Geometry check sheet. Reference: the model listing, model coordinates, mm. A direction names the side the tool comes from. Round coordinates to 2 decimals unless told otherwise and drop trailing zeros. Write each loop counter-clockwise with the first axis right and the second up, starting at its lowest first coordinate (ties: lowest second). Pieces come first, ordered by that corner, then holes. Notation, with made-up numbers: (3.25, -29.75) - (23.25, -29.75) arc R19 ccw to (23.25, -8.75) - close; hole circle Ø11 at (-1.75, 78.5). An arc over 180 degrees is marked (long way). Return JSON: item names as keys, results as strings.
```python
from build123d import *

# Parameters (mm, degrees)
ESQUISSE1_R             = 25.4
BOSS_EXTRU_1_DEPTH      = 25
ESQUISSE6_R             = 1.55
ENL_V_MAT_EXTRU_4_DEPTH = 6
ESQUISSE8_R             = 25.4
BOSS_EXTRU_3_DEPTH      = 10
ESQUISSE9_R             = 1.5
ENL_V_MAT_EXTRU_5_DEPTH = 10


with BuildPart() as part:
    # Esquisse1 → Boss.-Extru.1 (new body)
    with BuildSketch(Plane.XY):
        with Locations((16.625210007, 7.108710486)):
            Circle(ESQUISSE1_R)
    extrude(amount=BOSS_EXTRU_1_DEPTH)

    # Esquisse6 → Enlèv. mat.-Extru.4 (cut)
    with BuildSketch(Plane(origin=(0, 0, 0), x_dir=(-1, 0, 0), z_dir=(0, 0, -1))):
        with Locations((-39.525210007, 7.108710486)):
            Circle(ESQUISSE6_R)
        with Locations((6.274789993, 7.108710486)):
            Circle(ESQUISSE6_R)
    extrude(amount=-ENL_V_MAT_EXTRU_4_DEPTH, mode=Mode.SUBTRACT)

    # Esquisse8 → Boss.-Extru.3 (add)
    with BuildSketch(Plane.XY.offset(25)):
        with Locations((16.625210007, 7.108710486)):
            Circle(ESQUISSE8_R)
    extrude(amount=BOSS_EXTRU_3_DEPTH)

    # Esquisse9 → Enlèv. mat.-Extru.5 (cut)
    with BuildSketch(Plane.XY.offset(35)):
        with Locations((16.625210007, 7.108710486)):
            Circle(ESQUISSE9_R)
        with Locations((21.905210007, 7.108710486)):
            Circle(ESQUISSE9_R)
        with Locations((27.185210007, 7.108710486)):
            Circle(ESQUISSE9_R)
        with Locations((32.465210007, 7.108710486)):
            Circle(ESQUISSE9_R)
        with Locations((37.745210007, 7.108710486)):
            Circle(ESQUISSE9_R)
        with Locations((11.345210007, 7.108710486)):
            Circle(ESQUISSE9_R)
        with Locations((6.065210007, 7.108710486)):
            Circle(ESQUISSE9_R)
        with Locations((0.785210007, 7.108710486)):
            Circle(ESQUISSE9_R)
        with Locations((-4.494789993, 7.108710486)):
            Circle(ESQUISSE9_R)
        with Locations((0.785210007, 17.668710486)):
            Circle(ESQUISSE9_R)
        with Locations((6.065210007, 17.668710486)):
            Circle(ESQUISSE9_R)
        with Locations((11.345210007, 17.668710486)):
            Circle(ESQUISSE9_R)
        with Locations((16.625210007, 17.668710486)):
            Circle(ESQUISSE9_R)
        with Locations((21.905210007, 17.668710486)):
            Circle(ESQUISSE9_R)
        with Locations((27.185210007, 17.668710486)):
            Circle(ESQUISSE9_R)
        with Locations((32.465210007, 17.668710486)):
            Circle(ESQUISSE9_R)
        with Locations((8.705210007, 12.388710486)):
            Circle(ESQUISSE9_R)
        with Locations((13.985210007, 12.388710486)):
            Circle(ESQUISSE9_R)
        with Locations((19.265210007, 12.388710486)):
            Circle(ESQUISSE9_R)
        with Locations((24.545210007, 12.388710486)):
            Circle(ESQUISSE9_R)
        with Locations((29.825210007, 12.388710486)):
            Circle(ESQUISSE9_R)
        with Locations((35.105210007, 12.388710486)):
            Circle(ESQUISSE9_R)
        with Locations((3.425210007, 12.388710486)):
            Circle(ESQUISSE9_R)
        with Locations((-1.854789993, 12.388710486)):
            Circle(ESQUISSE9_R)
        with Locations((13.985210007, 22.948710486)):
            Circle(ESQUISSE9_R)
        with Locations((19.265210007, 22.948710486)):
            Circle(ESQUISSE9_R)
        with Locations((24.545210007, 22.948710486)):
            Circle(ESQUISSE9_R)
        with Locations((13.985210007, 28.228710486)):
            Circle(ESQUISSE9_R)
        with Locations((19.265210007, 28.228710486)):
            Circle(ESQUISSE9_R)
        with Locations((24.545210007, 28.228710486)):
            Circle(ESQUISSE9_R)
        with Locations((8.705210007, 22.948710486)):
            Circle(ESQUISSE9_R)
        with Locations((8.705210007, 28.228710486)):
            Circle(ESQUISSE9_R)
        with Locations((29.825210007, 22.948710486)):
            Circle(ESQUISSE9_R)
        with Locations((3.425210007, 22.948710486)):
            Circle(ESQUISSE9_R)
        with Locations((35.105210007, 1.828710486)):
            Circle(ESQUISSE9_R)
        with Locations((29.825210007, 1.828710486)):
            Circle(ESQUISSE9_R)
        with Locations((24.545210007, 1.828710486)):
            Circle(ESQUISSE9_R)
        with Locations((19.265210007, 1.828710486)):
            Circle(ESQUISSE9_R)
        with Locations((13.985210007, 1.828710486)):
            Circle(ESQUISSE9_R)
        with Locations((8.705210007, 1.828710486)):
            Circle(ESQUISSE9_R)
        with Locations((3.425210007, 1.828710486)):
            Circle(ESQUISSE9_R)
        with Locations((-1.854789993, 1.828710486)):
            Circle(ESQUISSE9_R)
        with Locations((0.785210007, -3.451289514)):
            Circle(ESQUISSE9_R)
        with Locations((6.065210007, -3.451289514)):
            Circle(ESQUISSE9_R)
        with Locations((11.345210007, -3.451289514)):
            Circle(ESQUISSE9_R)
        with Locations((16.625210007, -3.451289514)):
            Circle(ESQUISSE9_R)
        with Locations((21.905210007, -3.451289514)):
            Circle(ESQUISSE9_R)
        with Locations((27.185210007, -3.451289514)):
            Circle(ESQUISSE9_R)
        with Locations((32.465210007, -3.451289514)):
            Circle(ESQUISSE9_R)
        with Locations((29.825210007, -8.731289514)):
            Circle(ESQUISSE9_R)
        with Locations((24.545210007, -8.731289514)):
            Circle(ESQUISSE9_R)
        with Locations((19.265210007, -8.731289514)):
            Circle(ESQUISSE9_R)
        with Locations((13.985210007, -8.731289514)):
            Circle(ESQUISSE9_R)
        with Locations((8.705210007, -8.731289514)):
            Circle(ESQUISSE9_R)
        with Locations((3.425210007, -8.731289514)):
            Circle(ESQUISSE9_R)
        with Locations((8.705210007, -14.011289514)):
            Circle(ESQUISSE9_R)
        with Locations((13.985210007, -14.011289514)):
            Circle(ESQUISSE9_R)
        with Locations((19.265210007, -14.011289514)):
            Circle(ESQUISSE9_R)
        with Locations((24.545210007, -14.011289514)):
            Circle(ESQUISSE9_R)
    extrude(amount=-ENL_V_MAT_EXTRU_5_DEPTH, mode=Mode.SUBTRACT)

    # Esquisse12 → Enlèvement de matière-Révolution1 (revolve, cut)
    with BuildSketch(Plane(origin=(16.625210007, 0, 0), x_dir=(0, 0, -1), z_dir=(1, 0, 0))):
        Polygon((0, 7.108710486), (0, 27.108710486), (-25, 30.108710486), (-25, 7.108710486), align=None)
    revolve(axis=Axis((16.625210007, 7.108710486, 25), (0, 0, -1)), mode=Mode.SUBTRACT)


solid = part.part
```
(1) Gauge pin test, flat ends, axial feed: pin 1 (1 mm diameter, centred on x = 21.5, z = 13.5, fed in from -Y); pin 2 (4 mm diameter, centred on x = 27.19, y = 17.67, fed in from -Z); pin 3 (4 mm diameter, centred on x = 28, z = 30.5, fed in from -Y); pin 4 (1.8 mm diameter, centred on x = 16.63, y = -3.45, fed in from -Z). Record the tip position at first contact, or that the pin passes through.
Response values:
{"pin 1": "stops at y = -17.91", "pin 2": "stops at z = 25", "pin 3": "stops at y = -16.5", "pin 4": "passes through"}
(2) Release check for a two-part mould opening along X. For faces 4 (the face through (36.49, 1.25, 30.07)), 5 (the face through (11.119, -17.687, 17.255)) record: pulls with the +X half, pulls with the -X half, needs draft (parallel to the pull), parting line crosses it, or undercut.
Response values:
{"face 4": "undercut", "face 5": "parting line crosses it"}
(3) Section check B-B, the plane x = 32. Give the number of separate pieces and of enclosed holes in the cut face, plus the area to 3 significant figures.
Response values:
{"separate pieces": "4", "enclosed holes": "0", "area": "580 mm^2"}
(4) Material ranges on line 1 along Y through (x, z) = (11, 27); line 2 along Z through (x, y) = (0, 4.5); line 3 along X through (y, z) = (-3.5, 21), recorded low to high. Write a range as [from, to].
Response values:
{"line 1": "y = [-17.66, -4.91], [-1.99, 5.65], [8.57, 16.21], [19.13, 31.88]", "line 2": "z = [25, 35]", "line 3": "x = [-6.45, -3.24], [36.49, 39.7]"}
(5) Section check A-A, the plane z = 21.5. Enter the section's corners in (x, y).
Response values:
{"outline": "circle Ø50.8 at (16.63, 7.11); hole circle Ø45.16 at (16.63, 7.11)"}
(6) Access from +Z, -Z, +X, -X, +Y, -Y to the whole of each face (thin tool, end or side, straight path). Record for faces 1 (the face through (-4.726, 7.177, 2.958)), 2 (the face through (20.407, -3.385, 30.07)), 3 (the face through (25, -15, 25)).
Response values:
{"face 1": "-Z", "face 2": "+Z, -Z", "face 3": "+Z"}
